Geometry: final body of the model. Coordinates: model frame, mm. Face numbers are marked on the shaded views. A direction names the side the tool comes from. Coordinates: 2 decimals unless noted, no trailing zeros. Loops run counter-clockwise (first coordinate to the right, second up) from the corner with the lowest first, then second, coordinate; pieces in that order, holes last. Notation, with made-up numbers: (20, 72.5) - (34, 72.5) arc R23 cw to (34, 97.5) - close; hole circle Ø4 at (-39, 4). An arc over 180 degrees is marked (long way). Return JSON: item names as keys, results as strings.
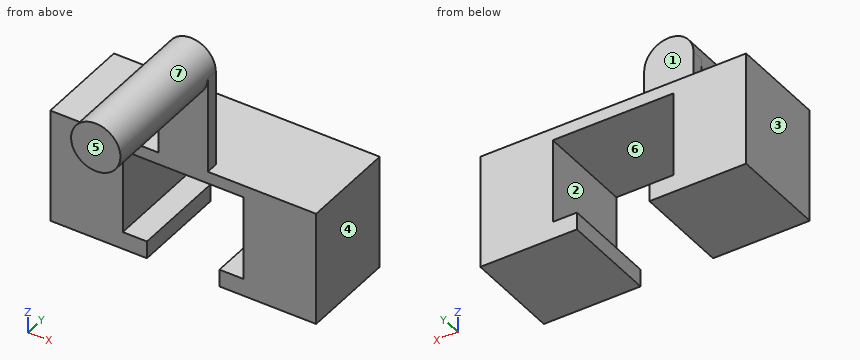
from build123d import *

# Parameters (mm, degrees)
SKETCH1_R           = 12.954
BOSS_EXTRUDE1_DEPTH = 76.2
SKETCH3_W           = 25.908
SKETCH3_H           = 50.8
BOSS_EXTRUDE3_DEPTH = 6.35
SKETCH7_W           = 63.5
SKETCH7_H           = 50.8
BOSS_EXTRUDE4_DEPTH = 6.35
SKETCH10_W          = 38.1
SKETCH10_H          = 50.8
BOSS_EXTRUDE6_DEPTH = 50.8
SKETCH11_W          = 50.8
SKETCH11_H          = 50.8
BOSS_EXTRUDE7_DEPTH = 9.144


with BuildPart() as part:
    # Sketch1 → Boss-Extrude1 (new body)
    with BuildSketch(Plane(origin=(0, 0, 0), x_dir=(1, 0, 0), z_dir=(0, 1, 0))):
        with Locations(Location((-1.734112165, 7.707165176, 0), (0, 0, 90))):
            Circle(SKETCH1_R)
    extrude(amount=BOSS_EXTRUDE1_DEPTH)

    # Sketch3 → Boss-Extrude3 (add)
    with BuildSketch(Plane(origin=(0, 76.2, 0), x_dir=(1, 0, 0), z_dir=(0, 1, 0))):
        with Locations((-1.734112165, 33.107165176)):
            Rectangle(SKETCH3_W, SKETCH3_H)
    extrude(amount=-BOSS_EXTRUDE3_DEPTH)

    # Sketch7 → Boss-Extrude4 (add)
    with BuildSketch(Plane(origin=(0, 0, -58.507165176), x_dir=(-1, 0, 0), z_dir=(0, 0, -1))):
        with Locations((1.734112165, 95.25)):
            Rectangle(SKETCH7_W, SKETCH7_H)
    extrude(amount=BOSS_EXTRUDE4_DEPTH)

    # Sketch10 → Boss-Extrude6 (add)
    with BuildSketch(Plane.XZ.offset(-69.85)):
        with Locations((-52.534112165, -83.907165176)):
            Rectangle(SKETCH10_W, SKETCH10_H)
        with Locations((49.065887835, -83.907165176)):
            Rectangle(SKETCH10_W, SKETCH10_H)
    extrude(amount=-BOSS_EXTRUDE6_DEPTH)

    # Sketch11 → Boss-Extrude7 (add)
    with BuildSketch(Plane(origin=(0, 0, -109.307165176), x_dir=(-1, 0, 0), z_dir=(0, 0, -1))):
        with Locations((-42.715887835, 95.25)):
            Rectangle(SKETCH11_W, SKETCH11_H)
        with Locations((46.184112165, 95.25)):
            Rectangle(SKETCH11_W, SKETCH11_H)
    extrude(amount=BOSS_EXTRUDE7_DEPTH)


solid = part.part
Item 1: Section query C-C, the plane x = -53. Return loops of the section in (y, z).
Worked out:
{"outline": "(69.85, -118.45) - (120.65, -118.45) - (120.65, -58.51) - (69.85, -58.51) - close"}
Item 2: First-contact query: pin 1 Ø14 at (x, y) = (-28.5, 89) entering from +Z; pin 2 Ø7 at (y, z) = (72, -32.5) entering from -X; pin 3 Ø2 at (x, z) = (47, -77.5) entering from -Y. Flat tips, straight axial feed; report the tip coordinate or a pass-through.
Worked out:
{"pin 1": "z = -58.51", "pin 2": "x = -14.69", "pin 3": "y = 69.85"}
Item 3: Section query A-A, the plane z = -91. Return loops of the section in (x, y).
Worked out:
{"outline": "(-71.58, 69.85) - (-33.48, 69.85) - (-33.48, 120.65) - (-71.58, 120.65) - close; (30.02, 69.85) - (68.12, 69.85) - (68.12, 120.65) - (30.02, 120.65) - close"}
Item 4: Section query B-B, the plane y = 98.5. Return loops of the section in (x, z), and give its area (3 significant figures).
Worked out:
{"outline": "(-71.58, -118.45) - (-20.78, -118.45) - (-20.78, -109.31) - (-33.48, -109.31) - (-33.48, -64.86) - (30.02, -64.86) - (30.02, -109.31) - (17.32, -109.31) - (17.32, -118.45) - (68.12, -118.45) - (68.12, -58.51) - (-71.58, -58.51) - close", "area": "5,200 mm^2"}
Item 5: Reachability of the marked faces 5, 6 and 7 from +Z, -Z, +X, -X, +Y, -Y: full face, straight path, thin tool, end or side. Return the list, or none.
Worked out:
{"face 5": "+Z, -Z, +X, -X, -Y", "face 6": "+Y, -Y", "face 7": "-Y"}
Item 6: Mould query, pull axis X, two halves, no side actions, for the marked faces 1, 2, 3 and 4. Classes: +X half, -X half, draft (parallel to the pull), parting line (faces both ways), or undercut.
Worked out:
{"face 1": "draft", "face 2": "undercut", "face 3": "-X half", "face 4": "+X half"}
Item 7: Section query D-D, the plane z = -14.5. Return loops of the section in (x, y), and give its area (3 significant figures).
Worked out:
{"outline": "(-14.69, 69.85) - (-12.76, 69.85) - (-12.76, 0) - (9.3, 0) - (9.3, 69.85) - (11.22, 69.85) - (11.22, 76.2) - (-14.69, 76.2) - close", "area": "1,710 mm^2"}
Item 8: Ray query, probe 1 along X at (y, z) = (107.5, -75.5); probe 2 along Y at (x, z) = (59, -99.5); probe 3 along Z at (x, y) = (-61, 81.5). Return the intervals inside material, ascending. Write a range as from..to.
Worked out:
{"probe 1": "-71.58..-33.48, 30.02..68.12", "probe 2": "69.85..120.65", "probe 3": "-118.45..-58.51"}
